Input: part model. Units: mm. Frame: model coordinates. A direction names the side the tool comes from. Coordinates: 2 decimals unless noted, no trailing zeros. Order: outer loops, then holes, each group sorted by start corner. A loop starts at its lowest first (then second) coordinate and runs counter-clockwise, first axis right, second up. Notation, with made-up numbers: (10.5, 85) -> (54.5, 85) arc R8 cw to (54.5, 90) -> close; hole circle Ø4 at (1, 87.25). An arc over 180 degrees is marked (long way). One line per question, with ' | ' between items.
```python
from build123d import *

# Parameters (mm, degrees)
SKETCH1_R               = 6.35
BOSS_EXTRUDE1_DEPTH     = 1.27
SKETCH2_R               = 4.95
SKETCH2_R_2             = 3.3782
BOSS_EXTRUDE2_DEPTH     = 16.49959986
SKETCH3_R               = 3.3782
CUT_EXTRUDE1_DEPTH      = 1
CUT_EXTRUDE1_DEPTH_BACK = 18.76959986


with BuildPart() as part:
    # Sketch1 → Boss-Extrude1 (new body)
    with BuildSketch(Plane(origin=(0, 0, 0), x_dir=(1, 0, 0), z_dir=(0, 1, 0))):
        Circle(SKETCH1_R)
    extrude(amount=BOSS_EXTRUDE1_DEPTH)

    # Sketch2 → Boss-Extrude2 (add)
    with BuildSketch(Plane(origin=(0, 1.27, 0), x_dir=(1, 0, 0), z_dir=(0, 1, 0))):
        Circle(SKETCH2_R)
        Circle(SKETCH2_R_2, mode=Mode.SUBTRACT)
    extrude(amount=BOSS_EXTRUDE2_DEPTH)

    # Sketch3 → Cut-Extrude1 (cut, two sides)
    with BuildSketch(Plane(origin=(0, 0, 0), x_dir=(-1, 0, 0), z_dir=(0, -1, 0))) as cut_extrude1_sk:
        Circle(SKETCH3_R)
    extrude(amount=CUT_EXTRUDE1_DEPTH, mode=Mode.SUBTRACT)
    extrude(cut_extrude1_sk.sketch, amount=-CUT_EXTRUDE1_DEPTH_BACK, mode=Mode.SUBTRACT)


solid = part.part
```
1. Mould query, pull axis X, two halves, no side actions, for faces 3 (the face through (-1.38, 0.63, 6.2)), 4 (the face through (2, 17.77, 3)), 5 (the face through (2.681, 8.76, 2.056)). Classes: released by +X, released by -X, zero draft, split by the parting line, or undercut.
Recorded:
face 3: split by the parting line | face 4: zero draft | face 5: undercut
2. Access query for faces 1 (the face through (3, 0, 3)), 2 (the face through (-2, 1.27, 5)). Directions: +Z, -Z, +X, -X, +Y, -Y. A direction counts if a zero-diameter tool reaches every point of the face in a straight line with its end or side. Return the directions, or none.
Recorded:
face 1: +Z, -Z, +X, -X, -Y | face 2: +Y
3. Pin query (flat end, axial travel): pin 1 Ø6 at (y, z) = (10.5, 2) entering from -X. Return the tip coordinate at first contact, or that it passes through.
Recorded:
pin 1: stops at x = -4.95
4. Cut plane A-A, the plane z = 0. Return loops of the section in (x, y).
Recorded:
outline: (-6.35, 0) -> (-3.38, 0) -> (-3.38, 17.77) -> (-4.95, 17.77) -> (-4.95, 1.27) -> (-6.35, 1.27) -> close; (3.38, 0) -> (6.35, 0) -> (6.35, 1.27) -> (4.95, 1.27) -> (4.95, 17.77) -> (3.38, 17.77) -> close
5. Ray query, line 1 (Z direction, x = 0, y = 2.75); line 2 (Y direction, x = 2.5, z = 5). Return the intervals inside material, ascending. Write a range as [from, to].
Recorded:
line 1: z = [-4.95, -3.38], [3.38, 4.95] | line 2: y = [0, 1.27]
6. Cut plane C-C, the plane y = 8.75. Return loops of the section in (x, z), and give its area (3 significant figures).
Recorded:
outline: circle Ø9.9 at (0, 0); hole circle Ø6.76 at (0, 0) | area: 41.1 mm^2
7. Cut plane B-B, the plane x = 0. Return loops of the section in (y, z).
Recorded:
outline: (0, -6.35) -> (1.27, -6.35) -> (1.27, -4.95) -> (17.77, -4.95) -> (17.77, -3.38) -> (0, -3.38) -> close; (0, 3.38) -> (17.77, 3.38) -> (17.77, 4.95) -> (1.27, 4.95) -> (1.27, 6.35) -> (0, 6.35) -> close
8. Cut plane D-D, the plane x = -4.5. Return loops of the section in (y, z).
Recorded:
outline: (0, -4.48) -> (1.27, -4.48) -> (1.27, -2.06) -> (17.77, -2.06) -> (17.77, 2.06) -> (1.27, 2.06) -> (1.27, 4.48) -> (0, 4.48) -> close
